Check sheet for the modelled part. Datum: model origin and axes. Units: mm. A direction names the side the tool comes from. Give positions to 0.01 mm unless a question says otherwise; leave off trailing zeros. Write each loop counter-clockwise with the first axis right and the second up, starting at its lowest first coordinate (ties: lowest second). Pieces come first, ordered by that corner, then holes.
Autodesk Inventor part; units mm, degrees
ref_plane "YZ Plane" through (0, 0, 0) normal (1, 0, 0) x (0, 1, 0)
ref_plane "XZ Plane" through (0, 0, 0) normal (0, 1, 0) x (-1, 0, 0)
ref_plane "XY Plane" through (0, 0, 0) normal (0, 0, 1) x (1, 0, 0)
sketch "スケッチ1" plane through (0, 0, 0) normal (0, 0, 1) x (1, 0, 0)
  circle A0 centre (0, 0) radius 2.5
  dimension "d0" = 5
extrude "押し出し1" add sketch "スケッチ1" along normal mid plane 51.4
sketch "スケッチ2" plane through (0, 0, 25.7) normal (0, 0, 1) x (1, 0, 0)
  circle A0 centre (0, 0) radius 10
  dimension "d3" = 20
extrude "押し出し2" add sketch "スケッチ2" against normal blind 2
sketch "スケッチ3" plane through (0, 0, -25.7) normal (0, 0, -1) x (-1, 0, 0)
  circle A0 centre (0, 0) radius 10
  dimension "d6" = 20
extrude "押し出し3" add sketch "スケッチ3" against normal blind 2
sketch "スケッチ4" plane through (0, 0, -25.7) normal (0, 0, -1) x (-1, 0, 0)
  point P0 (0, 0)
  point P1 (7, 0)
  point P2 (4.9497, 4.9497)
  point P3 (0, 7)
  point P4 (-4.9497, 4.9497)
  point P5 (-7, 0)
  point P6 (-4.9497, -4.9497)
  point P7 (0, -7)
  point P8 (4.9497, -4.9497)
  dimension "d9" = 7
  dimension "d12" = 360
hole "穴1" at (-7, 0, -25.7) at (-4.9497, 4.9497, -25.7) at (0, 7, -25.7) at (4.9497, 4.9497, -25.7) at (7, 0, -25.7) at (4.9497, -4.9497, -25.7) at (0, -7, -25.7) at (-4.9497, -4.9497, -25.7) direction (0, 0, 1) diameter 1 end through all
properties part number "サーボパーツ2"
1) Sectioned sample at A-A on y = 0. Record the boundary of the cut face in (x, z).
2) Scan lines: L1, parallel to Y at x = 0, z = 24.3; L2, parallel to Z at x = -2, y = 6; L3, parallel to X at y = 7, z = -24.75. Record each from-to range of solid material in increasing order.
3) Gauge pin test, flat ends, axial feed: pin 1 (1.5 mm diameter, centred on y = 4.5, z = 4.5, fed in from -X); pin 2 (1 mm diameter, centred on y = 2, z = -9.5, fed in from -X); pin 3 (5 mm diameter, centred on x = -1, z = -12, fed in from +Y); pin 4 (5 mm diameter, centred on x = -3, z = -3.5, fed in from +Y). Record the tip position at first contact, or that the pin passes through.
4) Access from +Z, -Z, +X, -X, +Y, -Y to the whole of each face (thin tool, end or side, straight path). Record for faces 1 (the flat face through (2, -2, 23.7)), 2 (the cylindrical face through (7.488, -0.108, -24.686)).
5) Sectioned sample at C-C on x = -3. Record the boundary of the cut face in (y, z).
6) Draft check along X on faces 3 (the flat face through (0, 0, 25.7)), 4 (the cylindrical face through (-0.15, 7.477, 24.714)), 5 (the cylindrical face through (-2.17, -9.76, 24.71)). Enter one of: +X half, -X half, draft (parallel to the pull), parting line (faces both ways), or undercut.
Answers below:
1. outline: (-10, -25.7) - (-7.5, -25.7) - (-7.5, -23.7) - (-10, -23.7) - close; (-10, 23.7) - (-7.5, 23.7) - (-7.5, 25.7) - (-10, 25.7) - close; (-6.5, -25.7) - (6.5, -25.7) - (6.5, -23.7) - (2.5, -23.7) - (2.5, 23.7) - (6.5, 23.7) - (6.5, 25.7) - (-6.5, 25.7) - (-6.5, 23.7) - (-2.5, 23.7) - (-2.5, -23.7) - (-6.5, -23.7) - close; (7.5, -25.7) - (10, -25.7) - (10, -23.7) - (7.5, -23.7) - close; (7.5, 23.7) - (10, 23.7) - (10, 25.7) - (7.5, 25.7) - close
2. L1: y = -10 to -7.5, -6.5 to 6.5, 7.5 to 10
2. L2: z = -25.7 to -23.7, 23.7 to 25.7
2. L3: x = -7.14 to -0.5, 0.5 to 7.14
3. pin 1: passes through
3. pin 2: stops at x = -2
3. pin 3: stops at y = 2.5
3. pin 4: stops at y = 2.45
4. face 1: none
4. face 2: +Z, -Z
5. outline: (-9.54, -25.7) - (9.54, -25.7) - (9.54, -23.7) - (-9.54, -23.7) - close; (-9.54, 23.7) - (9.54, 23.7) - (9.54, 25.7) - (-9.54, 25.7) - close
6. face 3: draft
6. face 4: undercut
6. face 5: parting line
